Design review of the part built by this model. Coordinates are the model's own, in mm. Face numbers are marked on the shaded views. Round coordinates to 2 decimals unless told otherwise and drop trailing zeros. Order: outer loops, then holes, each group sorted by start corner. A loop starts at its lowest first (then second) coordinate and runs counter-clockwise, first axis right, second up.
from build123d import *

# Parameters (mm, degrees)
SKETCH1_W           = 18
SKETCH1_H           = 30
BOSS_EXTRUDE1_DEPTH = 9
SKETCH2_W           = 12.5
SKETCH2_H           = 5.1
CUT_EXTRUDE1_DEPTH  = 10
FILLET1_R           = 4.5


with BuildPart() as part:
    # Sketch1 → Boss-Extrude1 (new body)
    with BuildSketch(Plane(origin=(0, 0, 0), x_dir=(1, 0, 0), z_dir=(0, 1, 0))):
        with Locations((9, 15)):
            Rectangle(SKETCH1_W, SKETCH1_H)
    extrude(amount=BOSS_EXTRUDE1_DEPTH)

    # Sketch2 → Cut-Extrude1 (cut)
    with BuildSketch(Plane(origin=(0, 0, -30), x_dir=(-1, 0, 0), z_dir=(0, 0, -1))):
        with Locations((-9, 4.5)):
            Rectangle(SKETCH2_W, SKETCH2_H)
    extrude(amount=-CUT_EXTRUDE1_DEPTH, mode=Mode.SUBTRACT)

    # Fillet1
    fillet1_edges = [part.edges().sort_by_distance(p)[0] for p in [
        (0, 0, -15),
        (0, 9, -15),
        (18, 0, -15),
        (18, 9, -15),
    ]]
    fillet(fillet1_edges, radius=FILLET1_R - 0.0001)  # a hair under: the kernel refuses the full size


solid = part.part
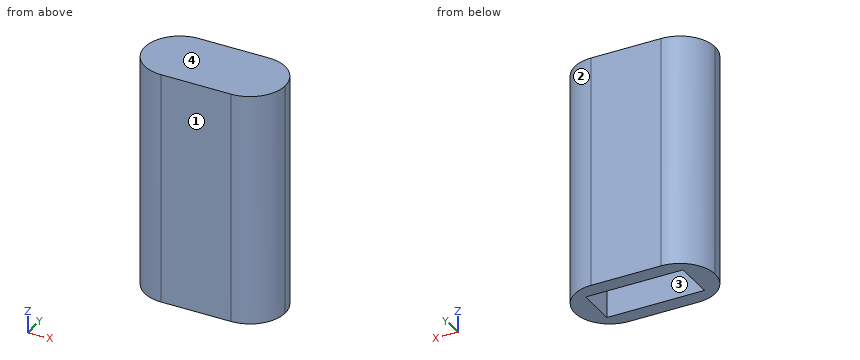
1) Clearance check with flat-ended pins moving along their axes: P1, Ø4, axis at y = 5, z = -25.5, coming from the -X side; P2, Ø1.5, axis at y = 3, z = -24, coming from the +X side; P3, Ø1.5, axis at x = 10.5, y = 3.5, coming from the -Z side. State where each tip first meets the part, or that it passes through.
Results:
P1: stops at x = 0
P2: stops at x = 17.94
P3: stops at z = -20
2) To check wall thickness, follow line 1 along Y through (x, z) = (10, -20.25); line 2 along Z through (x, y) = (12, 5.5); line 3 along X through (y, z) = (7.75, -6.75). State the ranges of each line that lie inside material, in increasing order.
Results:
line 1: y = 0 to 1.95, 7.05 to 9
line 2: z = -20 to 0
line 3: x = 1.39 to 16.61
3) Take a section at B-B on x = 6.75. Give the boundary of the cut face in (y, z).
Results:
outline: (0, -30) - (1.95, -30) - (1.95, -20) - (7.05, -20) - (7.05, -30) - (9, -30) - (9, 0) - (0, 0) - close
4) The part is to be moulded in two halves that separate along Y. For the marked faces 1, 2, 3 and 4, say which applies: released by +Y, released by -Y, zero draft, split by the parting line, or undercut.
Results:
face 1: released by -Y
face 2: released by +Y
face 3: undercut
face 4: zero draft
5) Take a section at D-D on y = 7.5. Give the boundary of the cut face in (x, z), plus the area to 3 significant figures.
Results:
outline: (1.15, -30) - (16.85, -30) - (16.85, 0) - (1.15, 0) - close
area: 471 mm2
